For this review, use the dimensioned drawing (mm, ordinates from the lowest corner) and the shaded views. A direction names the side the tool comes from. Coordinates: 2 decimals unless noted, no trailing zeros. Loops run counter-clockwise (first coordinate to the right, second up) from the corner with the lowest first, then second, coordinate; pieces in that order, holes last.
1. Take a section at D-D, the plane y = 5.6. State the section outline as (x, z) points (1 decimal).
2. Take a section at A-A, the plane z = 0.9. State the section outline as (x, y) points.
3. Take a section at C-C, the plane x = 32.5. State the section outline as (y, z) points.
4. Machinability: for the marked faces 1 and 2, which of the approach directions +Z, -Z, +X, -X, +Y, -Y give a long, thin tool a straight path to every point of the face, cutting with its end or side? Answer none if there is none.
5. Take a section at B-B, the plane y = 17.5. State the section outline as (x, z) points (1 decimal).
6. To check wall thickness, follow probe 1 along Y at (x, z) = (21, 2.3) (1 decimal); probe 2 along X at (y, z) = (8, 1.75) (1 decimal); probe 3 along Y at (x, z) = (35, 1.6) (1 decimal). State the ranges of each line that lie inside material, in increasing order.
7. Clearance check with flat-ended pins moving along their axes: P1, Ø3.5, axis at x = 21.5, y = 31, coming from the -Z side; P2, Ø3.5, axis at x = 4.5, y = 6, coming from the -Z side. State where each tip first meets the part, or that it passes through.
8. Mouldability with a two-part tool opening along X and no side actions: class the marked faces 3, 4 and 5 as pulls with the +X half, pulls with the -X half, needs draft (parallel to the pull), parting line crosses it, or undercut.
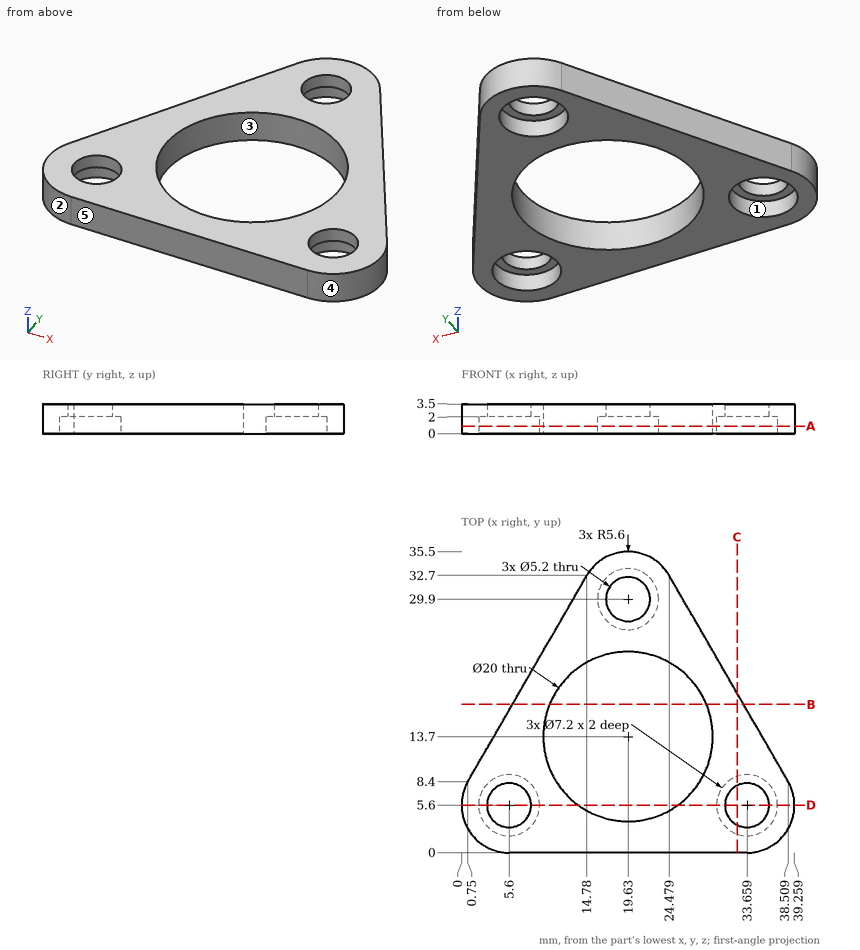
Results list:
1. outline: (0, 0) - (2, 0) - (2, 2) - (3, 2) - (3, 3.5) - (0, 3.5) - close; (8.2, 2) - (9.2, 2) - (9.2, 0) - (13.8, 0) - (13.8, 3.5) - (8.2, 3.5) - close; (25.5, 0) - (30.1, 0) - (30.1, 2) - (31.1, 2) - (31.1, 3.5) - (25.5, 3.5) - close; (36.3, 2) - (37.3, 2) - (37.3, 0) - (39.3, 0) - (39.3, 3.5) - (36.3, 3.5) - close
2. outline: (0.75, 8.4) arc R5.6 ccw to (5.6, 0) - (33.66, 0) arc R5.6 ccw to (38.51, 8.4) - (24.48, 32.7) arc R5.6 ccw to (14.78, 32.7) - close; hole circle Ø7.2 at (5.6, 5.6); hole circle Ø20 at (19.63, 13.7); hole circle Ø7.2 at (19.63, 29.9); hole circle Ø7.2 at (33.66, 5.6)
3. outline: (0, 0) - (2.19, 0) - (2.19, 2) - (3.27, 2) - (3.27, 3.5) - (0, 3.5) - close; (7.93, 2) - (9.01, 2) - (9.01, 0) - (18.81, 0) - (18.81, 3.5) - (7.93, 3.5) - close
4. face 1: -Z
4. face 2: +Z, -Z, -X
5. outline: (6, 0) - (10.4, 0) - (10.4, 3.5) - (6, 3.5) - close; (28.9, 0) - (33.3, 0) - (33.3, 3.5) - (28.9, 3.5) - close
6. probe 1: y = 0 to 3.8, 23.6 to 27.7, 32.1 to 35.3
6. probe 2: x = 0.5 to 2.9, 8.3 to 11.4, 27.8 to 31, 36.3 to 38.7
6. probe 3: y = 0.2 to 2.3, 8.9 to 14.5
7. P1: stops at z = 0
7. P2: stops at z = 2
8. face 3: undercut
8. face 4: pulls with the +X half
8. face 5: needs draft
